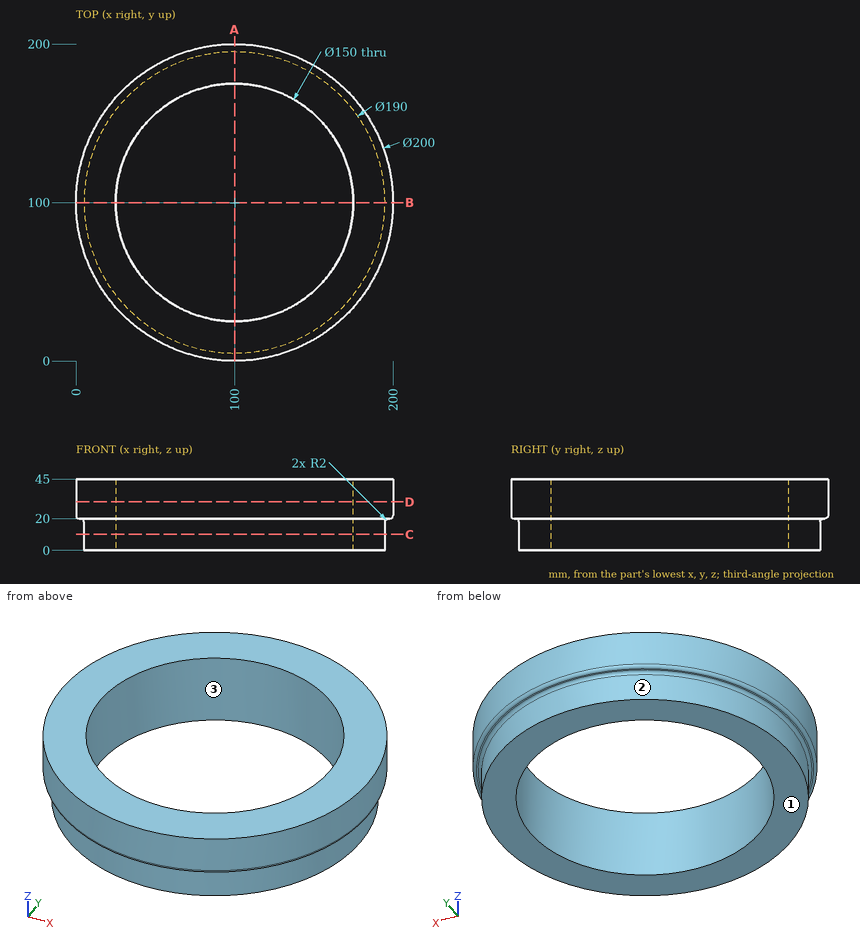
Drawing for the job (mm, zero at the part's lowest x, y, z). Give positions to 0.01 mm unless a question says otherwise; leave off trailing zeros. Order: outer loops, then holes, each group sorted by start corner. A loop starts at its lowest first (then second) coordinate and runs counter-clockwise, first axis right, second up. Notation, with made-up numbers: M 22.25,-39 L 45.25,-39 A14 ccw 45.25,-24 Z; hole C 62,39.5 d2. An arc over 180 degrees is marked long. Put each result on its own line as item: value.
Item 1: Slice it at A-A, the plane x = 100. Write the cut outline in (y, z), plus the area to 3 significant figures.
From the geometry:
outline: M 0,22 A2 ccw 2,20 L 3,20 A2 cw 5,18 L 5,0 L 25,0 L 25,45 L 0,45 Z; M 175,0 L 195,0 L 195,18 A2 cw 197,20 L 198,20 A2 ccw 200,22 L 200,45 L 175,45 Z
area: 2,050 mm2
Item 2: Slice it at C-C, the plane z = 10. Write the cut outline in (x, y).
From the geometry:
outline: C 100,100 d190; hole C 100,100 d150
Item 3: Flat gauge pins, fed straight in: pin 1 Ø2 at (y, z) = (69, 13.5) entering from -X; pin 2 Ø3 at (x, z) = (37, 30.5) entering from +Y; pin 3 Ø1 at (x, z) = (49, 37.5) entering from -Y. Where does each tip first touch, or does it go through?
From the geometry:
pin 1: stops at x = 9.86
pin 2: stops at y = 178.85
pin 3: stops at y = 13.69
Item 4: Probe line 1 (Y direction, x = 100, z = 25); line 2 (Y direction, x = 100, z = 12). List the from-to ranges inside material, lowest first. Write a range as [from, to].
From the geometry:
line 1: y = [0, 25], [175, 200]
line 2: y = [5, 25], [175, 195]
Item 5: Two-plate mould, pull along Y, no slides. Class the marked faces 1, 2 and 3: +Y half, -Y half, draft (parallel to the pull), parting line (faces both ways), or undercut.
From the geometry:
face 1: draft
face 2: parting line
face 3: undercut
Item 6: Slice it at D-D, the plane z = 30.5. Write the cut outline in (x, y), plus the area to 3 significant figures.
From the geometry:
outline: C 100,100 d200; hole C 100,100 d150
area: 13,700 mm2
